Autodesk Inventor part; units mm, degrees
ref_plane "YZ Plane" through (0, 0, 0) normal (1, 0, 0) x (0, 1, 0)
ref_plane "XZ Plane" through (0, 0, 0) normal (0, 1, 0) x (-1, 0, 0)
ref_plane "XY Plane" through (0, 0, 0) normal (0, 0, 1) x (1, 0, 0)
sketch "Skizze1" plane through (0, 0, 0) normal (0, 1, 0) x (-1, 0, 0)
  line L0 (-2, 0) -> (-7.5, 0)
  line L1 (-9.5, -2) -> (-9.5, -7.5)
  line L2 (-7.5, -9.5) -> (-2, -9.5)
  line L3 (0, -7.5) -> (0, -2)
  arc A0 (-2, -9.5) -> (0, -7.5) centre (-2, -7.5) ccw
  arc A1 (-9.5, -7.5) -> (-7.5, -9.5) centre (-7.5, -7.5) ccw
  arc A2 (-7.5, 0) -> (-9.5, -2) centre (-7.5, -2) ccw
  arc A3 (0, -2) -> (-2, 0) centre (-2, -2) ccw
  point P0 (0, 0)
  point P1 (-9.5, -9.5)
  point P2 (-9.5, 0)
  point P3 (0, -9.5)
  dimension "d0" = 9.5
  dimension "d1" = 9.5
  dimension "d2" = 2
extrude "Extrusion1" add sketch "Skizze1" along normal blind 5
sketch "Skizze2" plane through (0, 5, 0) normal (0, 1, 0) x (1, 0, 0)
  arc A0 (7.5, 0) -> (9.5, 2) centre (7.5, 2) ccw
  line L0 (9.5, 2) -> (9.5, 7.5)
  arc A1 (9.5, 7.5) -> (7.5, 9.5) centre (7.5, 7.5) ccw
  line L1 (7.5, 9.5) -> (2, 9.5)
  arc A2 (2, 9.5) -> (0, 7.5) centre (2, 7.5) ccw
  line L2 (0, 7.5) -> (0, 2)
  arc A3 (0, 2) -> (2, 0) centre (2, 2) ccw
  line L3 (2, 0) -> (7.5, 0)
  circle A4 centre (4.75, 4.75) radius 3.5
  line L4 (9.5, 2) -> (9.5, 7.5)
  arc A5 (7.5, -2) -> (11.5, 2) centre (7.5, 2) ccw
  line L5 (7.5, -2) -> (2, -2)
  arc A6 (-2, 2) -> (2, -2) centre (2, 2) ccw
  line L6 (-2, 2) -> (-2, 7.5)
  arc A7 (2, 11.5) -> (-2, 7.5) centre (2, 7.5) ccw
  line L7 (2, 11.5) -> (7.5, 11.5)
  arc A8 (11.5, 7.5) -> (7.5, 11.5) centre (7.5, 7.5) ccw
  line L8 (11.5, 7.5) -> (11.5, 2)
  point P0 (0, 0)
  point P1 (9.5, 4.75)
  point P2 (4.75, 9.5)
  dimension "d5" = 7
  dimension "d6" = 2
extrude "Extrusion2" add sketch "Skizze2" along normal blind 2 contours L3 A3 L2 A2 L1 A1 L0 A0 | L5 A6 L6 A7 L7 A8 L8 A5
sketch "Skizze3" plane through (4.75, 5, -4.75) normal (0, 1, 0) x (1, 0, 0)
  circle A0 centre (0, 0) radius 3.5
  line L0 (-3.3541, 1) -> (3.3541, 1)
  line L1 (3.3541, 1) -> (3.3541, -1)
  line L2 (3.3541, -1) -> (-3.3541, -1)
  line L3 (-3.3541, -1) -> (-3.3541, 1)
  circle A1 centre (0, 0) radius 3.5
  point P0 (-4.75, -4.75)
  dimension "d9" = 2
extrude "Extrusion3" cut sketch "Skizze3" against normal through all contours L1 L2 L3 L0
properties part number "led_stand"
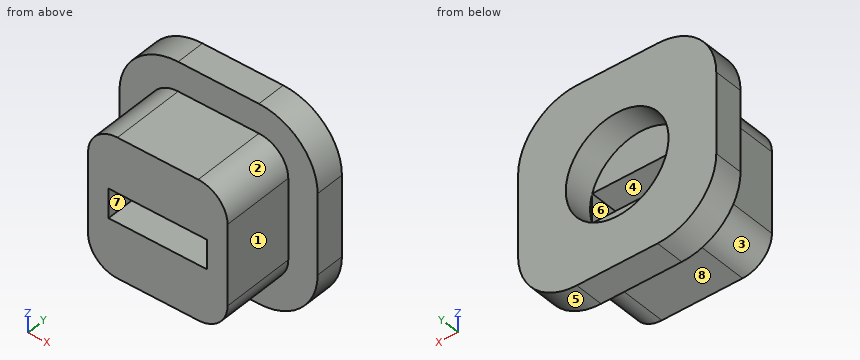
For this review, take the finished solid that the model builds, in its own axes (mm). Face numbers are marked on the shaded views. A direction names the side the tool comes from. Coordinates: 2 decimals unless noted, no trailing zeros. Write each loop counter-clockwise with the first axis right and the second up, starting at its lowest first coordinate (ties: lowest second). Pieces come first, ordered by that corner, then holes. Notation, with made-up numbers: (-1, 84.25) - (54, 84.25) arc R9 cw to (54, 98.25) - close; hole circle Ø3 at (-1.75, 81.25). An arc over 180 degrees is marked (long way). Answer in a Markdown table with one row per item. Add a question column.
Q1. For P1, Ø1, axis at y = 5.5, z = -0.5, coming from the -X side; P2, Ø1.6, axis at y = 3, z = -5, coming from the +X side; P3, Ø1.2, axis at x = 3.5, z = -3, coming from the +Y side, all flat-tipped, find the tip position at first contact; note any pin that passes through.
Q2. We need section A-A, the plane z = -4.75. State the section outline as (x, y) points, and give its area (3 significant figures).
Q3. We need section D-D, the plane z = -9. State the section outline as (x, y) points.
Q4. Tool access review of the marked faces 1, 2, 3 and 4: name each direction out of +Z, -Z, +X, -X, +Y, -Y from which nothing blocks a thin tool from reaching the whole face with its end or side.
Q5. Draft analysis for pull direction X (two halves, no side actions). For the marked faces 5, 6, 7 and 8, state which applies: +X half, -X half, draft (parallel to the pull), parting line (faces both ways), or undercut.
Q6. We need section B-B, the plane x = 4.75. State the section outline as (y, z) points.
Q7. We need section C-C, the plane y = 4. State the section outline as (x, z) points, and give its area (3 significant figures).
Q8. For probe 1 along X at (y, z) = (6.05, -4.75); probe 2 along Z at (x, y) = (4.75, 6.15); probe 3 along Z at (x, y) = (4.75, 1.5), list the stretches that pass through material, from the lowest coordinate up.
Answer list:
| question | item | result |
|---|---|---|
| 1 | P1 | stops at x = -1.87 |
| 1 | P2 | stops at x = 9.5 |
| 1 | P3 | stops at y = 5 |
| 2 | outline | (-2, 5) - (0, 5) - (0, 0) - (1.4, 0) - (1.4, 5) - (1.25, 5) - (1.25, 7) - (-2, 7) - close; (8.1, 0) - (9.5, 0) - (9.5, 5) - (11.5, 5) - (11.5, 7) - (8.25, 7) - (8.25, 5) - (8.1, 5) - close |
| 2 | area | 27.0 mm2 |
| 3 | outline | (-1.71, 5) - (0.68, 5) - (0.68, 0) - (8.82, 0) - (8.82, 5) - (11.21, 5) - (11.21, 7) - (-1.71, 7) - close |
| 4 | face 1 | +Z, -Z, +X, -Y |
| 4 | face 2 | +Z, +X, -Y |
| 4 | face 3 | -Z, -X, -Y |
| 4 | face 4 | +Y, -Y |
| 5 | face 5 | +X half |
| 5 | face 6 | undercut |
| 5 | face 7 | undercut |
| 5 | face 8 | draft |
| 6 | outline | (0, -9.5) - (5, -9.5) - (5, -11.5) - (7, -11.5) - (7, -8.25) - (5, -8.25) - (5, -5.75) - (0, -5.75) - close; (0, -3.75) - (5, -3.75) - (5, -1.25) - (7, -1.25) - (7, 2) - (5, 2) - (5, 0) - (0, 0) - close |
| 7 | outline | (0, -7.5) arc R2 ccw to (2, -9.5) - (7.5, -9.5) arc R2 ccw to (9.5, -7.5) - (9.5, -2) arc R2 ccw to (7.5, 0) - (2, 0) arc R2 ccw to (0, -2) - close; hole (1.4, -5.75) - (8.1, -5.75) - (8.1, -3.75) - (1.4, -3.75) - close |
| 7 | area | 73.4 mm2 |
| 8 | probe 1 | x = -2 to 1.25, 8.25 to 11.5 |
| 8 | probe 2 | z = -11.5 to -8.25, -1.25 to 2 |
| 8 | probe 3 | z = -9.5 to -5.75, -3.75 to 0 |
